Build history of the part. All positions in model axes, mm. Face numbers are marked on the shaded views. A direction names the side the tool comes from. Give positions to 0.01 mm unless a question says otherwise; leave off trailing zeros.
1) Wall check: line 1 (Y direction, x = 2.5, z = -1); line 2 (Y direction, x = 9.25, z = 4); line 3 (Z direction, x = 15.5, y = 15). Give the ranges that are in metal, low to high.
2) Flat gauge pins, fed straight in: P1, Ø1.5, axis at x = 5.5, z = -2, coming from the +Y side; P2, Ø2, axis at x = 4, z = -2, coming from the -Y side; P3, Ø1.5, axis at x = 3.5, y = 8, coming from the -Z side. Where does each tip first touch, or does it go through?
3) Band-saw the part on A-A on z = -2.5. State how many separate pieces and enclosed holes the cut face has, then the cut area to 3 significant figures.
4) 3-axis set-ups, long thin cutter, end or side, ignore diameter. For the marked faces 1 and 2: which of +Z, -Z, +X, -X, +Y, -Y reach the whole face in a straight line?
```python
from build123d import *

# Parameters (mm, degrees)
EXTRUDE_1_DEPTH = 17.5
SKETCH_6_W      = 0.51
SKETCH_6_H      = 0.25
EXTRUDE_2_DEPTH = 4.89


with BuildPart() as part:
    # 草图2 → 凸台-拉伸1 (new body)
    with BuildSketch(Plane(origin=(0, 0, 0), x_dir=(0, 0, -1), z_dir=(1, 0, 0))):
        Polygon((-3.442512479, 20.118929979), (0.792082517, 20.118929979), (0.792082517, 19.034466272), (0, 19.034466272), (0, 0.792082517), (0.792082517, 0.792082517), (0.792082517, 0), (0, 0), (-3.442512479, 0), (-3.79285667, 1.095795152), (-5.283117125, 1.682856003), (-5.283117125, 3.191302286), (-3.79285667, 3.850153416), (-3.79285667, 16.026820243), (-5.283117125, 16.71396292), (-5.283117125, 18.019534007), (-3.937694697, 18.484803601), align=None)
    extrude(amount=EXTRUDE_1_DEPTH)

    # 草图5 → 旋转8 (revolve)
    with BuildSketch(Plane.XY.offset(2.89285667)):
        with BuildLine():
            Line((0, 10.068929979), (17.5, 10.068929979))
            Line((17.5, 10.068929979), (17.5, 11.490689909))
            ThreePointArc((17.5, 11.490689909), (15.277289221, 12.591913923), (13.2, 11.236182744))
            ThreePointArc((13.2, 11.236182744), (10.975, 12.596281432), (8.75, 11.236182744))
            ThreePointArc((8.75, 11.236182744), (6.517271028, 12.596269485), (4.292994354, 11.222403449))
            ThreePointArc((4.292994354, 11.222403449), (2.215086636, 12.56500204), (0, 11.463338455))
            Line((0, 11.463338455), (0, 10.068929979))
        make_face()
    revolve(axis=Axis((0, 10.068929979, 2.89285667), (1, 0, 0)))

    # 草图6 → 凸台-拉伸2 (add)
    with BuildSketch(Plane(origin=(0, 0, 0), x_dir=(-1, 0, 0), z_dir=(0, 0, -1))):
        with Locations((-12.56, 17.709464989)):
            Rectangle(SKETCH_6_W, SKETCH_6_H)
        with Locations((-15.1, 17.709464989)):
            Rectangle(SKETCH_6_W, SKETCH_6_H)
        with Locations((-10.02, 17.709464989)):
            Rectangle(SKETCH_6_W, SKETCH_6_H)
        with Locations((-7.48, 17.709464989)):
            Rectangle(SKETCH_6_W, SKETCH_6_H)
        with Locations((-4.94, 17.709464989)):
            Rectangle(SKETCH_6_W, SKETCH_6_H)
        with Locations((-2.4, 17.709464989)):
            Rectangle(SKETCH_6_W, SKETCH_6_H)
        with Locations((-15.1, 2.409464989)):
            Rectangle(SKETCH_6_W, SKETCH_6_H)
        with Locations((-12.56, 2.409464989)):
            Rectangle(SKETCH_6_W, SKETCH_6_H)
        with Locations((-10.02, 2.409464989)):
            Rectangle(SKETCH_6_W, SKETCH_6_H)
        with Locations((-7.48, 2.409464989)):
            Rectangle(SKETCH_6_W, SKETCH_6_H)
        with Locations((-4.94, 2.409464989)):
            Rectangle(SKETCH_6_W, SKETCH_6_H)
        with Locations((-2.4, 2.409464989)):
            Rectangle(SKETCH_6_W, SKETCH_6_H)
    extrude(amount=EXTRUDE_2_DEPTH)


solid = part.part
```
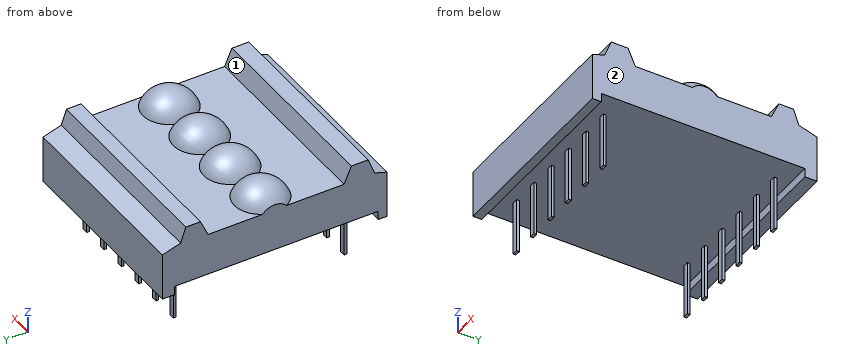
Findings below:
1. line 1: y = 2.28 to 2.53, 17.58 to 17.83
1. line 2: y = 1.18 to 3.76, 8.6 to 11.53, 16.12 to 18.46
1. line 3: z = 0 to 3.79
2. P1: stops at y = 17.83
2. P2: stops at y = 2.28
2. P3: stops at z = 0
3. separate pieces: 12
3. enclosed holes: 0
3. area: 1.53 mm2
4. face 1: +Z, +X, -X
4. face 2: +Z, -Z, +X, +Y, -Y
